The listing builds one solid part. Answer for the finished solid, in the listing's coordinates (mm). Round coordinates to 2 decimals unless told otherwise and drop trailing zeros. Write each loop counter-clockwise with the first axis right and the second up, starting at its lowest first coordinate (ties: lowest second). Pieces come first, ordered by that corner, then holes.
from build123d import *

# Parameters (mm, degrees)
CYLINDER875_R          = 1.6
CYLINDER875_DEPTH      = 20
CYLINDER875_ROLL_ANGLE = 90
CYLINDER876_R          = 1.6
CYLINDER876_DEPTH      = 20
CYLINDER876_ROLL_ANGLE = 90
CYLINDER874_R          = 1.6
CYLINDER874_DEPTH      = 20
CYLINDER874_ROLL_ANGLE = 90
BOX544_W               = 30
BOX544_H               = 3.75
BOX544_DEPTH           = 14


with BuildPart() as cylinder1036:
    # Cylinder875 → Cylinder875 (new body)
    with BuildSketch(Plane.XY):
        Circle(CYLINDER875_R)
    extrude(amount=CYLINDER875_DEPTH)


with BuildPart() as cylinder1036_1:
    # Cylinder875 roll: moved
    add(cylinder1036.part.rotate(Axis((0, 0, 0), (1, 0, 0)), CYLINDER875_ROLL_ANGLE))


with BuildPart() as cylinder1036_2:
    # Cylinder875 placement: moved
    add(cylinder1036_1.part.moved(Location((49.5, 56.5, -13))))


with BuildPart() as cylinder1037:
    # Cylinder876 → Cylinder876 (new body)
    with BuildSketch(Plane.XY):
        Circle(CYLINDER876_R)
    extrude(amount=CYLINDER876_DEPTH)


with BuildPart() as cylinder1037_1:
    # Cylinder876 roll: moved
    add(cylinder1037.part.rotate(Axis((0, 0, 0), (1, 0, 0)), CYLINDER876_ROLL_ANGLE))


with BuildPart() as cylinder1037_2:
    # Cylinder876 placement: moved
    add(cylinder1037_1.part.moved(Location((37, 56.5, -11))))


with BuildPart() as fusion562:
    # Cylinder874 → Cylinder874 (new body)
    with BuildSketch(Plane.XY):
        Circle(CYLINDER874_R)
    extrude(amount=CYLINDER874_DEPTH)


with BuildPart() as fusion562_1:
    # Cylinder874 roll: moved
    add(fusion562.part.rotate(Axis((0, 0, 0), (1, 0, 0)), CYLINDER874_ROLL_ANGLE))


with BuildPart() as fusion562_2:
    # Cylinder874 placement: moved
    add(fusion562_1.part.moved(Location((28.5, 56.5, -11))))

    # Fusion562: union Cylinder1036, Cylinder1037
    add(cylinder1036_2.part)
    add(cylinder1037_2.part)


with BuildPart() as obj1:
    # Box544 → Box544 (new body)
    with BuildSketch(Plane(origin=(23.5, 49.75, -18), x_dir=(1, 0, 0), z_dir=(0, 0, 1))):
        with Locations((15, 1.875)):
            Rectangle(BOX544_W, BOX544_H)
    extrude(amount=BOX544_DEPTH)

    # Cut668: cut Fusion562
    add(fusion562_2.part, mode=Mode.SUBTRACT)


solid = obj1.part
1. Section B-B on x = 37 is taken. Determine the outline of the cut face in (y, z), plus the area to 3 significant figures.
Geometry says:
outline: (49.75, -18) - (53.5, -18) - (53.5, -12.6) - (49.75, -12.6) - close; (49.75, -9.4) - (53.5, -9.4) - (53.5, -4) - (49.75, -4) - close
area: 40.5 mm2
2. Section A-A on z = -13 is taken. Determine the outline of the cut face in (x, y), plus the area to 4 significant figures.
Geometry says:
outline: (23.5, 49.75) - (47.9, 49.75) - (47.9, 53.5) - (23.5, 53.5) - close; (51.1, 49.75) - (53.5, 49.75) - (53.5, 53.5) - (51.1, 53.5) - close
area: 100.5 mm2
3. Section C-C on z = -11 is taken. Determine the outline of the cut face in (x, y).
Geometry says:
outline: (23.5, 49.75) - (26.9, 49.75) - (26.9, 53.5) - (23.5, 53.5) - close; (30.1, 49.75) - (35.4, 49.75) - (35.4, 53.5) - (30.1, 53.5) - close; (38.6, 49.75) - (53.5, 49.75) - (53.5, 53.5) - (38.6, 53.5) - close
4. Straight lines are drawn through the part: line 1 along X through (y, z) = (51.8, -11); line 2 along Z through (x, y) = (49.5, 52.55); line 3 along X through (y, z) = (52.1, -13). For each, find the intervals that lie inside material, in ascending order.
Geometry says:
line 1: x = 23.5 to 26.9, 30.1 to 35.4, 38.6 to 53.5
line 2: z = -18 to -14.6, -11.4 to -4
line 3: x = 23.5 to 47.9, 51.1 to 53.5
5. Section D-D on y = 51.2 is taken. Determine the outline of the cut face in (x, z), plus the area to 3 significant figures.
Geometry says:
outline: (23.5, -18) - (53.5, -18) - (53.5, -4) - (23.5, -4) - close; hole circle Ø3.2 at (28.5, -11); hole circle Ø3.2 at (37, -11); hole circle Ø3.2 at (49.5, -13)
area: 396 mm2
6. For a pull along Z with two mould halves and no side action, classify faces 1 (the face through (38, 52, -4)), 2 (the face through (23.5, 52, -11)), 3 (the face through (38, 52, -18)), 4 (the face through (36.65, 51.65, -12.56)) as released by +Z, released by -Z, zero draft, split by the parting line, or undercut.
Geometry says:
face 1: released by +Z
face 2: zero draft
face 3: released by -Z
face 4: undercut
7. Given pin 1 (2.5 mm diameter, centred on x = 37, z = -11, fed in from +Y), flat-ended and moving along its own axis, determine where the tip first touches the part or whether it passes through.
Geometry says:
pin 1: passes through
